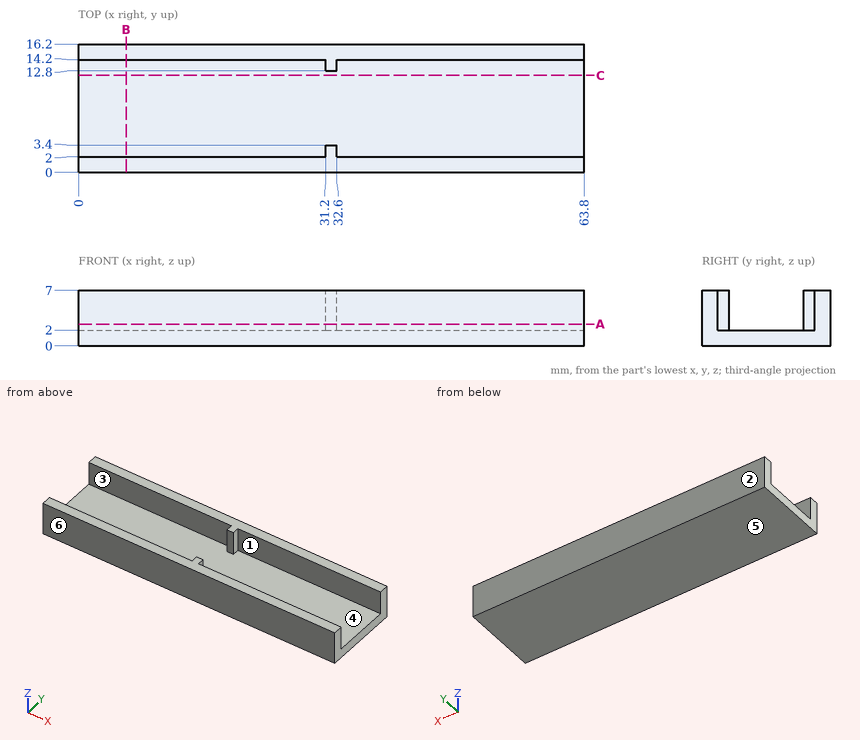
Design review of the part shown in the three views and the two pictorial views. Dimensions are in mm from the part's minimum x, y and z. A direction names the side the tool comes from. Round coordinates to 2 decimals unless told otherwise and drop trailing zeros. Order: outer loops, then holes, each group sorted by start corner. A loop starts at its lowest first (then second) coordinate and runs counter-clockwise, first axis right, second up. Notation, with made-up numbers: (64.25, 31) - (97.25, 31) arc R18 ccw to (97.25, 61) - close; hole circle Ø2 at (-35.5, 16). An arc over 180 degrees is marked (long way). One line per question, with ' | ' between items.
Item 1: Machinability: for the marked faces 1 and 2, which of the approach directions +Z, -Z, +X, -X, +Y, -Y give a long, thin tool a straight path to every point of the face, cutting with its end or side? Answer none if there is none.
Checks:
face 1: +Z, +X | face 2: +Z, -Z, +X, -X, +Y
Item 2: Take a section at C-C, the plane y = 12.25. Write out the cut boundary in (x, z).
Checks:
outline: (0, 0) - (63.8, 0) - (63.8, 2) - (0, 2) - close
Item 3: For P1, Ø0.7, axis at y = 13.5, z = 3.5, coming from the +X side; P2, Ø3, axis at x = 17, z = 1.5, coming from the -Y side; P3, Ø0.7, axis at y = 2.5, z = 5.5, coming from the -X side; P4, Ø5, axis at x = 33.5, y = 6, coming from the +Z side, all flat-tipped, find the tip position at first contact; note any pin that passes through.
Checks:
P1: x = 32.6 | P2: y = 0 | P3: x = 31.2 | P4: z = 2
Item 4: Wall thickness on line 1 (Y direction, x = 54.5, z = 6.75); line 2 (X direction, y = 13.25, z = 4); line 3 (Z direction, x = 28, y = 9.25): over which ranges is each line inside the solid? List them lowest first. Write a range as [from, to].
Checks:
line 1: [0, 2], [14.2, 16.2] | line 2: [31.2, 32.6] | line 3: [0, 2]
Item 5: Draft analysis for pull direction Y (two halves, no side actions). For the marked faces 3, 4, 5 and 6, state which applies: +Y half, -Y half, draft (parallel to the pull), parting line (faces both ways), or undercut.
Checks:
face 3: undercut | face 4: undercut | face 5: draft | face 6: -Y half
Item 6: Take a section at A-A, the plane z = 2.75. Write out the cut boundary in (x, y), then the cut area to 3 significant figures.
Checks:
outline: (0, 0) - (63.8, 0) - (63.8, 2) - (32.6, 2) - (32.6, 3.4) - (31.2, 3.4) - (31.2, 2) - (0, 2) - close; (0, 14.2) - (31.2, 14.2) - (31.2, 12.8) - (32.6, 12.8) - (32.6, 14.2) - (63.8, 14.2) - (63.8, 16.2) - (0, 16.2) - close | area: 259 mm²
Item 7: Take a section at B-B, the plane x = 6. Write out the cut boundary in (y, z), then the cut area to 3 significant figures.
Checks:
outline: (0, 0) - (16.2, 0) - (16.2, 7) - (14.2, 7) - (14.2, 2) - (2, 2) - (2, 7) - (0, 7) - close | area: 52.4 mm²
